Source: CAD feature listing. Evaluate the final solid. Frame: model axes, mm. A direction names the side the tool comes from. Give positions to 0.01 mm unless a question says otherwise; leave off trailing zeros. Loops run counter-clockwise (first coordinate to the right, second up) from the corner with the lowest first, then second, coordinate; pieces in that order, holes last. Notation, with made-up numbers: M 55,48 L 62,48 A11 ccw 62,64 Z; hole C 78.25,1.5 d11. An arc over 180 degrees is marked long. Put each result on its own line as item: value.
from build123d import *

# Parameters (mm, degrees)
SKETCH_1_W          = 35
SKETCH_1_H          = 39
EXTRUDE_1_DEPTH     = 8
SKETCH_2_R          = 1.65
CUT_EXTRUDE_1_DEPTH = 12
SKETCH_5_R          = 5.5
CUT_EXTRUDE_3_DEPTH = 5
CUT_EXTRUDE_5_DEPTH = 5
SKETCH_8_R          = 1.5
CUT_EXTRUDE_6_DEPTH = 5
CUT_EXTRUDE_START   = -12
SKETCH_9_R          = 1.65
CUT_EXTRUDE_7_DEPTH = 12


with BuildPart() as part:
    # 草图1 → 凸台-拉伸1 (new body)
    with BuildSketch(Plane(origin=(0, 0, 0), x_dir=(1, 0, 0), z_dir=(0, 1, 0))):
        Rectangle(SKETCH_1_W, SKETCH_1_H)
    extrude(amount=EXTRUDE_1_DEPTH)

    # 草图2 → 切除-拉伸1 (cut)
    with BuildSketch(Plane(origin=(0, 0, -19.5), x_dir=(-1, 0, 0), z_dir=(0, 0, -1))):
        with Locations((12.5, 4)):
            Circle(SKETCH_2_R)
        with Locations(Location((-12.5, 4, 0), (0, 0, 180))):
            Circle(SKETCH_2_R)
    extrude(amount=-CUT_EXTRUDE_1_DEPTH, mode=Mode.SUBTRACT)

    # 草图5 → 切除-拉伸3 (cut)
    with BuildSketch(Plane(origin=(0, 0, 0), x_dir=(1, 0, 0), z_dir=(0, 1, 0))):
        with Locations(Location((0, 4, 0), (0, 0, 270))):
            Circle(SKETCH_5_R)
    extrude(amount=CUT_EXTRUDE_3_DEPTH, mode=Mode.SUBTRACT)

    # 草图7 → 切除-拉伸5 (cut)
    with BuildSketch(Plane.XZ):
        with BuildLine():
            Line((1.5, -11), (1.5, -9))
            Line((1.5, -9), (-1.5, -9))
            Line((-1.5, -9), (-1.5, -11))
            ThreePointArc((-1.5, -11), (0, -12.5), (1.5, -11))
        make_face()
        with BuildLine():
            Line((-7, -5.5), (-5, -5.5))
            Line((-5, -5.5), (-5, -2.5))
            Line((-5, -2.5), (-7, -2.5))
            ThreePointArc((-7, -2.5), (-8.5, -4), (-7, -5.5))
        make_face()
        with BuildLine():
            Line((-1.5, 3), (-1.5, 1))
            Line((-1.5, 1), (1.5, 1))
            Line((1.5, 1), (1.5, 3))
            ThreePointArc((1.5, 3), (0, 4.5), (-1.5, 3))
        make_face()
        with BuildLine():
            Line((7, -2.5), (5, -2.5))
            Line((5, -2.5), (5, -5.5))
            Line((5, -5.5), (7, -5.5))
            ThreePointArc((7, -5.5), (8.5, -4), (7, -2.5))
        make_face()
    extrude(amount=-CUT_EXTRUDE_5_DEPTH, mode=Mode.SUBTRACT)

    # 草图8 → 切除-拉伸6 (cut)
    with BuildSketch(Plane.XZ.offset(-5)):
        with Locations(Location((0, -11, 0), (0, 0, 180))):
            Circle(SKETCH_8_R)
        with Locations(Location((7, -4, 0), (0, 0, 90))):
            Circle(SKETCH_8_R)
        with Locations((0, 3)):
            Circle(SKETCH_8_R)
        with Locations(Location((-7, -4, 0), (0, 0, 90))):
            Circle(SKETCH_8_R)
    extrude(amount=-CUT_EXTRUDE_6_DEPTH, mode=Mode.SUBTRACT)

    # 草图9 → 切除-拉伸7 (cut)
    with BuildSketch(Plane.XY.offset(19.5).offset(CUT_EXTRUDE_START)):
        with Locations(Location((-12.5, 4, 0), (0, 0, 180))):
            Circle(SKETCH_9_R)
        with Locations((12.5, 4)):
            Circle(SKETCH_9_R)
    extrude(amount=CUT_EXTRUDE_7_DEPTH, mode=Mode.SUBTRACT)


solid = part.part
1. Access query for faces 4 (the flat face through (-12, 4, 7.5)), 5 (the flat face through (-1.5, 2, -10)), 6 (the flat face through (12, 4, -7.5)). Directions: +Z, -Z, +X, -X, +Y, -Y. A direction counts if a zero-diameter tool reaches every point of the face in a straight line with its end or side. Return the directions, or none.
Found:
face 4: +Z
face 5: -Y
face 6: -Z
2. Section query C-C (y = 7). Output: boundary loops of the cut face in (x, z).
Found:
outline: M -17.5,-19.5 L 17.5,-19.5 L 17.5,19.5 L -17.5,19.5 Z; hole C -7,-4 d3; hole C 0,-11 d3; hole C 0,3 d3; hole C 7,-4 d3
3. Draft query along Z for faces 1 (the flat face through (0, 4, 19.5)), 2 (the flat face through (0, 5, -4)), 3 (the flat face through (-12, 4, -7.5)). Return one class per face: pulls with the +Z half, pulls with the -Z half, needs draft (parallel to the pull), parting line crosses it, or undercut.
Found:
face 1: pulls with the +Z half
face 2: undercut
face 3: pulls with the -Z half
4. Section query B-B (x = 0). Output: boundary loops of the cut face in (y, z).
Found:
outline: M 0,-19.5 L 8,-19.5 L 8,-12.5 L 0,-12.5 Z; M 0,4.5 L 8,4.5 L 8,19.5 L 0,19.5 Z; M 5,-9.5 L 8,-9.5 L 8,1.5 L 5,1.5 Z
5. Section query A-A (z = -12). Output: boundary loops of the cut face in (x, y).
Found:
outline: M -17.5,0 L -1.12,0 L -1.12,8 L -17.5,8 Z; M 1.12,0 L 17.5,0 L 17.5,8 L 1.12,8 Z; hole C -12.5,4 d3.3; hole C 12.5,4 d3.3
6. Section query D-D (z = 2). Output: boundary loops of the cut face in (x, y), plus the area to 3 significant figures.
Found:
outline: M -17.5,0 L -1.5,0 L -1.5,5 L -1.12,5 L -1.12,8 L -17.5,8 Z; M 1.12,5 L 1.5,5 L 1.5,0 L 17.5,0 L 17.5,8 L 1.12,8 Z
area: 258 mm^2
7. Material intervals for line 1 (Z direction, x = 0, y = 7.5); line 2 (Z direction, x = 7, y = 7.1); line 3 (Y direction, x = 12.5, z = -13.75), sorted ascending. Write a range as from..to.
Found:
line 1: -19.5..-12.5, -9.5..1.5, 4.5..19.5
line 2: -19.5..-5.5, -2.5..19.5
line 3: 0..2.35, 5.65..8
8. Contact query for flat-ended pins moving along their axis: P1, Ø1, axis at x = 13, y = 3.5, coming from the +Z side; P2, Ø2.5, axis at x = 0, z = -11, coming from the -Y side. Output: stop coordinate, or through.
Found:
P1: z = 7.5
P2: through
